```python
from build123d import *

# Parameters (mm, degrees)
SKETCH2_R               = 2.286
SKETCH2_R_2             = 2.54
BOSS_EXTRUDE1_DEPTH     = 6.35
SKETCH3_W               = 50.8
SKETCH3_H               = 27.94
BOSS_EXTRUDE2_DEPTH     = 6.35
SKETCH5_W               = 50.8
SKETCH5_H               = 6.35
BOSS_EXTRUDE3_DEPTH     = 6.35
CUT_EXTRUDE1_DEPTH      = 38.1
CUT_EXTRUDE1_DEPTH_BACK = 2.54
SKETCH6_R               = 6.35
BOSS_EXTRUDE4_START     = 6.35
SKETCH7_W               = 50.8
SKETCH7_H               = 6.35
SKETCH7_R               = 2.54
BOSS_EXTRUDE4_DEPTH     = 6.35
CUT_EXTRUDE2_DEPTH      = 3.175
SKETCH9_R               = 2.564291027
CUT_EXTRUDE3_DEPTH      = 127
SKETCH11_W              = 3.175
SKETCH11_H              = 37.465
CUT_EXTRUDE4_DEPTH      = 1.5875
SKETCH16_R              = 5.842
CUT_EXTRUDE7_DEPTH      = 3.81
SKETCH17_W              = 19.191430616
SKETCH17_H              = 21.182889484
CUT_EXTRUDE8_DEPTH      = 87.593141183
BOSS_EXTRUDE5_REACH     = 76.336


with BuildPart() as part:
    # Sketch2 → Boss-Extrude1 (new body)
    with BuildSketch(Plane(origin=(0, 0, 0), x_dir=(1, 0, 0), z_dir=(0, 1, 0))):
        Polygon((0, 0), (50.8, 0), (50.8, -57.15), align=None)
        with Locations(Location((38.1, -6.35, 0), (0, 0, 270))):
            Circle(SKETCH2_R, mode=Mode.SUBTRACT)
        with Locations(Location((38.1, -31.75, 0), (0, 0, 270))):
            Circle(SKETCH2_R_2, mode=Mode.SUBTRACT)
        with Locations(Location((10.699885901, -4.857157432, 0), (0, 0, 270))):
            Circle(SKETCH2_R_2, mode=Mode.SUBTRACT)
    extrude(amount=BOSS_EXTRUDE1_DEPTH)



with BuildPart() as body_2:
    # Sketch3 → Boss-Extrude2 (new body)
    with BuildSketch(Plane(origin=(0, 0, 0), x_dir=(-1, 0, 0), z_dir=(0, 0, -1))):
        with Locations((-25.4, -13.97)):
            Rectangle(SKETCH3_W, SKETCH3_H)
    extrude(amount=BOSS_EXTRUDE2_DEPTH)


with BuildPart() as part_1:
    add(part.part)

    add(body_2.part)  # Boss-Extrude3 merges body 2
    # Sketch5 → Boss-Extrude3 (add)
    with BuildSketch(Plane(origin=(0, 6.35, 0), x_dir=(1, 0, 0), z_dir=(0, 1, 0))):
        with Locations((25.4, 3.175)):
            Rectangle(SKETCH5_W, SKETCH5_H)
    extrude(amount=-BOSS_EXTRUDE3_DEPTH)

    # Sketch6 → Cut-Extrude1 (cut, two sides: drawn at the far end of the back side and taken through both)
    with BuildSketch(Plane.XZ.offset(-CUT_EXTRUDE1_DEPTH_BACK)):
        with Locations(Location((38.1, 6.35, 0), (0, 0, 270))):
            Circle(SKETCH6_R)
    extrude(amount=CUT_EXTRUDE1_DEPTH + CUT_EXTRUDE1_DEPTH_BACK, mode=Mode.SUBTRACT)

    # Sketch7 → Boss-Extrude4 (add)
    # profile 1 of 2: a face of its own
    with BuildSketch(Plane.XZ.offset(27.94).offset(BOSS_EXTRUDE4_START)):
        with Locations((25.4, -3.175)):
            Rectangle(SKETCH7_W, SKETCH7_H)
    # profile 2 of 2: a face of its own
    with BuildSketch(Plane.XZ.offset(27.94).offset(BOSS_EXTRUDE4_START)):
        Polygon((50.8, 57.15), (0, 0), (50.8, 0), align=None)
        with Locations(Location((38.1, 31.75, 0), (0, 0, 90))):
            Circle(SKETCH7_R, mode=Mode.SUBTRACT)
    extrude(amount=-BOSS_EXTRUDE4_DEPTH)

    # Sketch8 → Cut-Extrude2 (cut)
    with BuildSketch(Plane(origin=(0, 6.35, 0), x_dir=(1, 0, 0), z_dir=(0, 1, 0))):
        Polygon((26.9875, 6.35), (49.2125, 6.35), (49.2125, -55.3640625), (26.9875, -30.3609375), align=None)
    extrude(amount=-CUT_EXTRUDE2_DEPTH, mode=Mode.SUBTRACT)

    # Sketch9 → Cut-Extrude3 (cut)
    with BuildSketch(Plane(origin=(0, 6.35, 0), x_dir=(1, 0, 0), z_dir=(0, 1, 0))):
        with Locations(Location((10.699885901, -4.857157432, 0), (0, 0, 90))):
            Circle(SKETCH9_R)
    extrude(amount=-CUT_EXTRUDE3_DEPTH, mode=Mode.SUBTRACT)

    # Sketch11 → Cut-Extrude4 (cut)
    with BuildSketch(Plane(origin=(0, 0, -6.35), x_dir=(-1, 0, 0), z_dir=(0, 0, -1))):
        with Locations((-38.1, -15.5575)):
            Rectangle(SKETCH11_W, SKETCH11_H)
    extrude(amount=-CUT_EXTRUDE4_DEPTH, mode=Mode.SUBTRACT)

    # Sketch16 → Cut-Extrude7 (cut)
    with BuildSketch(Plane.XZ.offset(34.29)):
        with Locations(Location((38.1, 31.75, 0), (0, 0, 270))):
            Circle(SKETCH16_R)
    extrude(amount=-CUT_EXTRUDE7_DEPTH, mode=Mode.SUBTRACT)

    # Sketch17 → Cut-Extrude8 (cut, through all)
    with BuildSketch(Plane(origin=(0, 6.35, 0), x_dir=(1, 0, 0), z_dir=(0, 1, 0))):
        with Locations((41.204284692, -46.558555258)):
            Rectangle(SKETCH17_W, SKETCH17_H)
        Polygon((3.992356435, -4.491400989), (14.833757424, 6.35), (0, 6.35), (0, 0), align=None)
    extrude(amount=-CUT_EXTRUDE8_DEPTH, mode=Mode.SUBTRACT)

    # Boss-Extrude5: up to this face of the body (flat: up to its plane)
    boss_extrude5_end = Plane(part_1.part.faces().sort_by_distance((32.258274594, -34.29, 11.14322166))[0])
    # Sketch18 → Boss-Extrude5 (add, up to the picked face)
    with BuildSketch(Plane(origin=(0, 6.35, 0), x_dir=(1, 0, 0), z_dir=(0, 1, 0)), mode=Mode.PRIVATE) as boss_extrude5_sk1:
        Polygon((14.833757424, 6.35), (-6.915485897, 6.35), (3.992356435, -4.491400989), align=None)
    boss_extrude5_tool1 = split(extrude(boss_extrude5_sk1.sketch, amount=-BOSS_EXTRUDE5_REACH, mode=Mode.PRIVATE), bisect_by=boss_extrude5_end, keep=Keep.BOTH, mode=Mode.PRIVATE)
    add(boss_extrude5_tool1.solids().sort_by(Axis((3.970209, 6.35, -2.7362), (0, -1, 0)))[0])


solid = part_1.part
```
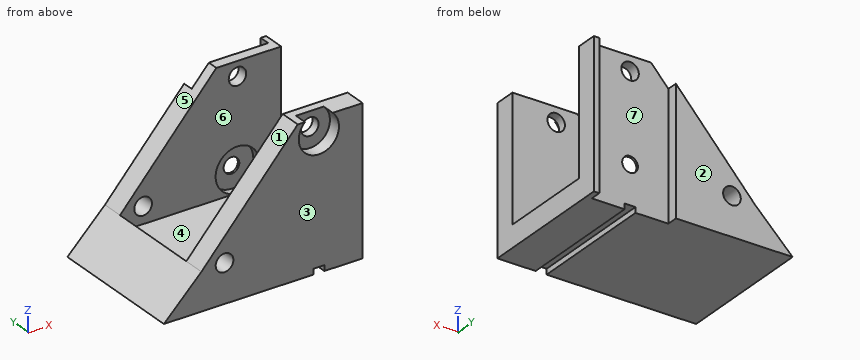
Source: CAD feature listing. Evaluate the final solid. Frame: model axes, mm. Face numbers are marked on the shaded views. A direction names the side the tool comes from. Coordinates: 2 decimals unless noted, no trailing zeros. Order: outer loops, then holes, each group sorted by start corner. A loop starts at its lowest first (then second) coordinate and runs counter-clockwise, first axis right, second up. Notation, with made-up numbers: M 40,-23.5 L 88,-23.5 A22 cw 88,1.5 Z; hole C 13,35 d1. An arc over 180 degrees is marked long. Write each question's results on one line, items separated by ' | '. Start each with the question number.
1) Section query B-B (x = 16). Return the cut outline in (y, z), plus the area to 3 significant figures.
2) Contact query for flat-ended pins moving along their axis: pin 1 Ø10 at (y, z) = (-2.5, 12.5) entering from -X; pin 2 Ø1.6 at (y, z) = (4.5, 20) entering from -X; pin 3 Ø15 at (x, z) = (38.1, 31.75) entering from +Y (3 decimals). Output: stop coordinate, or through.
3) Section query D-D (y = -9). Return the cut outline in (x, z).
4) Access query for the marked faces 5, 6 and 7. Directions: +Z, -Z, +X, -X, +Y, -Y. A direction counts if a zero-diameter tool reaches every point of the face in a straight line with its end or side. Return the directions, or none.
5) Section query A-A (z = 31.75). Give the number of separate pieces and of enclosed holes in the cut face, plus the area to 3 significant figures.
6) Line query: line 1 (Z direction, x = 38.1, y = 2.25); line 2 (X direction, y = 2.7, z = 6.35); line 3 (Y direction, x = 28, z = 19.5) (3 decimals). Output: solid intervals per line, ascending. Write a range as from..to.
7) Draft query along Y for the marked faces 1, 2, 3 and 4. Return one class per face: released by +Y, released by -Y, zero draft, split by the parting line, or undercut.
Answers:
1) outline: M -34.29,-6.35 L 6.35,-6.35 L 6.35,18 L 0,18 L 0,0 L -27.94,0 L -27.94,18 L -34.29,18 Z | area: 487 mm^2
2) pin 1: stops at x = 7.26 | pin 2: stops at x = 17.07 | pin 3: stops at y = 3.175
3) outline: M -6.92,-6.35 L 36.51,-6.35 L 36.51,-4.76 L 39.69,-4.76 L 39.69,-6.35 L 50.8,-6.35 L 50.8,0 L 8.48,0 L 3.99,4.49 Z
4) face 5: +Z, -X, +Y, -Y | face 6: +Z, +X | face 7: +Z, -Z, +Y
5) separate pieces: 4 | enclosed holes: 0 | area: 147 mm^2
6) line 1: z = -4.76..0, 12.7..29.21, 34.29..35.97 | line 2: x = 5.64..8.61, 12.78..35.81, 40.39..50.8 | line 3: y = -34.29..-27.94, 0..3.175
7) face 1: zero draft | face 2: released by +Y | face 3: released by -Y | face 4: undercut
